from build123d import *

# Parameters (mm, degrees)
ESQUISSE1_W             = 42
ESQUISSE1_H             = 25
BOSS_EXTRU_1_DEPTH      = 39
ESQUISSE2_W             = 10
ESQUISSE2_H             = 3
ENL_V_MAT_EXTRU_1_DEPTH = 10
ESQUISSE3_W             = 4
ESQUISSE3_H             = 3
ENL_V_MAT_EXTRU_2_DEPTH = 10


with BuildPart() as part:
    # Esquisse1 → Boss.-Extru.1 (new body)
    with BuildSketch(Plane.XY):
        Rectangle(ESQUISSE1_W, ESQUISSE1_H)
    extrude(amount=BOSS_EXTRU_1_DEPTH)

    # Esquisse2 → Enlèv. mat.-Extru.1 (cut)
    with BuildSketch(Plane(origin=(0, 0, 0), x_dir=(-1, 0, 0), z_dir=(0, 0, -1))):
        with Locations((11, -0.28777271)):
            Rectangle(ESQUISSE2_W, ESQUISSE2_H)
    extrude(amount=-ENL_V_MAT_EXTRU_1_DEPTH, mode=Mode.SUBTRACT)

    # Esquisse3 → Enlèv. mat.-Extru.2 (cut)
    with BuildSketch(Plane(origin=(-16, 0, 0), x_dir=(0, 0, -1), z_dir=(1, 0, 0))):
        with Locations((-8, -0.28777271)):
            Rectangle(ESQUISSE3_W, ESQUISSE3_H)
    extrude(amount=-ENL_V_MAT_EXTRU_2_DEPTH, mode=Mode.SUBTRACT)


solid = part.part
Work out the finished part from the listing and answer in its coordinate system (mm). A direction names the side the tool comes from. Give positions to 0.01 mm unless a question says otherwise; leave off trailing zeros. Order: outer loops, then holes, each group sorted by start corner. A loop starts at its lowest first (then second) coordinate and runs counter-clockwise, first axis right, second up. Notation, with made-up numbers: (71, 32.25) -> (119, 32.25) arc R36 ccw to (119, 67.25) -> close; hole circle Ø11 at (11, 54). An arc over 180 degrees is marked (long way). One line per item, written item: value.
Item 1: A straight line is drawn through the part: probe 1 along X at (y, z) = (-1.75, 5.5). Find the intervals that lie inside material, in ascending order.
Answer sheet:
probe 1: -21 to -16, -6 to 21
Item 2: A tool of negligible diameter and unlimited length cuts with its end or side. For faces 1 (the flat face through (-13, 0, 10)), 2 (the flat face through (-16, 0, 3)), 3 (the flat face through (-12, -1.788, 5)), from which of +Z, -Z, +X, -X, +Y, -Y can it reach the whole face along a straight path? Write none if from no direction.
Answer sheet:
face 1: -X
face 2: -Z
face 3: none
Item 3: Determine the mould class of faces 4 (the flat face through (21, 0, 19)), 5 (the flat face through (-21, 0, 19)), 6 (the flat face through (-12, 1.212, 5)), 7 (the flat face through (0, 12.5, 19)) for opening direction X: released by +X, released by -X, zero draft, split by the parting line, or undercut.
Answer sheet:
face 4: released by +X
face 5: released by -X
face 6: undercut
face 7: zero draft
Item 4: A flat-ended cylindrical pin translates along its axis: P1, Ø1.5, axis at y = -0.5, z = 7, coming from the -X side. Find the tip coordinate at first contact, or state that the pin passes through.
Answer sheet:
P1: x = -6
Item 5: Find section A-A, the plane x = -7. Give the vertices of the cut face in (y, z), plus the area to 3 significant figures.
Answer sheet:
outline: (-12.5, 0) -> (-1.79, 0) -> (-1.79, 10) -> (1.21, 10) -> (1.21, 0) -> (12.5, 0) -> (12.5, 39) -> (-12.5, 39) -> close
area: 945 mm²
